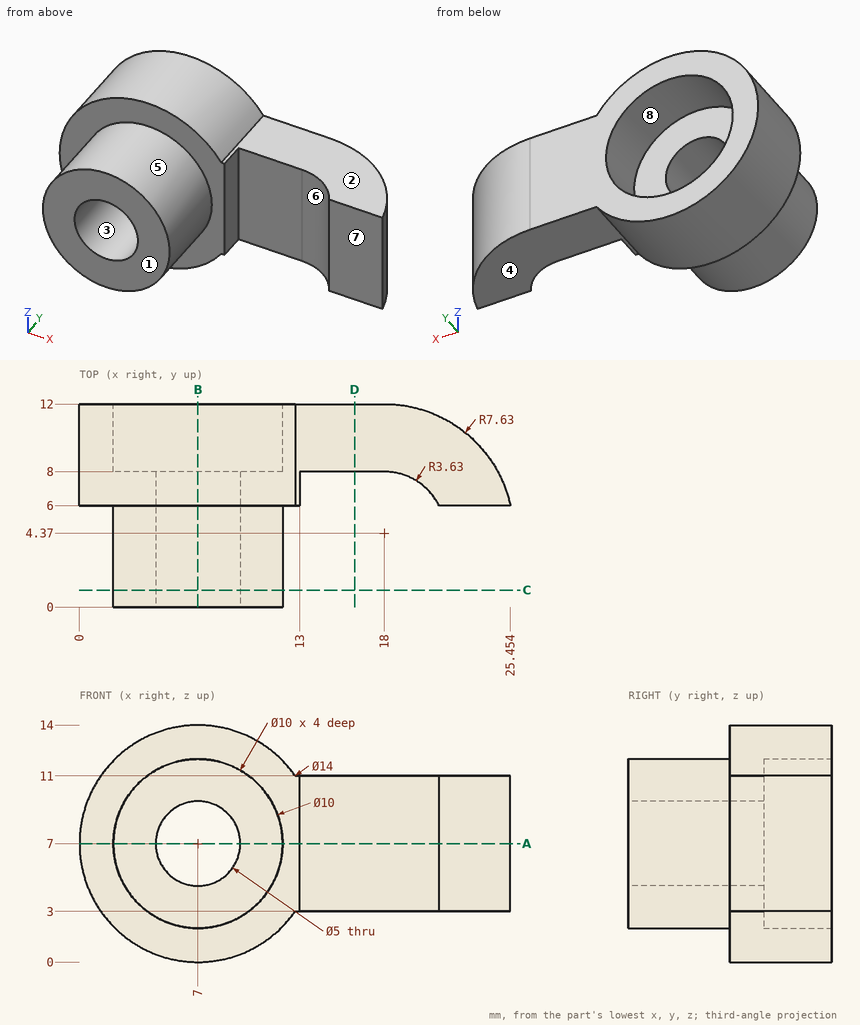
Study the drawing (mm; zero at the part's minimum x, y, z) and answer. A direction names the side the tool comes from. Coordinates: 2 decimals unless noted, no trailing zeros. Write each loop counter-clockwise with the first axis right and the second up, starting at its lowest first coordinate (ties: lowest second). Pieces come first, ordered by that corner, then holes. Notation, with made-up numbers: M 64.25,0 L 75.25,0 A11 ccw 75.25,9 Z; hole C -1.75,72.25 d3. An arc over 180 degrees is marked long. Use one line per item in the form item = value.
Item 1: Find section B-B, the plane x = 7. Give the vertices of the cut face in (y, z), plus the area to 3 significant figures.
Model answer:
outline = M 0,2 L 6,2 L 6,0 L 12,0 L 12,2 L 8,2 L 8,4.5 L 0,4.5 Z; M 0,9.5 L 8,9.5 L 8,12 L 12,12 L 12,14 L 6,14 L 6,12 L 0,12 Z
area = 64.0 mm2
Item 2: Find section D-D, the plane x = 16.25. Give the vertices of the cut face in (y, z).
Model answer:
outline = M 8,3 L 12,3 L 12,11 L 8,11 Z
Item 3: The mould has two halves that part along Z. Classify the marked faces 1, 2, 3 and 4: released by +Z, released by -Z, zero draft, split by the parting line, or undercut.
Model answer:
face_1 = zero draft
face_2 = released by +Z
face_3 = undercut
face_4 = released by -Z
Item 4: Find section C-C, the plane y = 1. Give the vertices of the cut face in (x, z).
Model answer:
outline = C 7,7 d10; hole C 7,7 d5
Item 5: Given P1, Ø6, axis at x = 7, z = 7, coming from the +Y side; P2, Ø6.5, axis at x = 18.5, y = 10.5, coming from the +Z side; P3, Ø1.3, axis at x = 23.5, z = 5.5, coming from the -Y side, each flat-ended and moving along its own axis, determine where each tip first touches the part or whether it passes through.
Model answer:
P1 = 8
P2 = 11
P3 = 6
Item 6: Find section A-A, the plane z = 7. Give the vertices of the cut face in (x, y).
Model answer:
outline = M 0,6 L 2,6 L 2,0 L 4.5,0 L 4.5,8 L 2,8 L 2,12 L 0,12 Z; M 9.5,0 L 12,0 L 12,6 L 13,6 L 13,8 L 18,8 A3.63 cw 21.24,6 L 25.45,6 A7.63 ccw 18,12 L 12,12 L 12,8 L 9.5,8 Z
Item 7: Find the intervals of material crossed by probe 1 along X at (y, z) = (10.55, 7) (1 decimal); probe 2 along Y at (x, z) = (9.25, 12.5); probe 3 along X at (y, z) = (10.5, 3.75), in increasing order.
Model answer:
probe_1 = 0 to 2, 12 to 22.5
probe_2 = 6 to 12
probe_3 = 0.8 to 3.2, 10.8 to 22.54
Item 8: For the marked faces 5, 6, 7 and 8, determine the directions among +Z, -Z, +X, -X, +Y, -Y from which every point of the face is accessible in a straight line to the end or side of a thin tool.
Model answer:
face_5 = -Y
face_6 = +Z, -Z, -Y
face_7 = +Z, -Z, +X, -Y
face_8 = +Y
